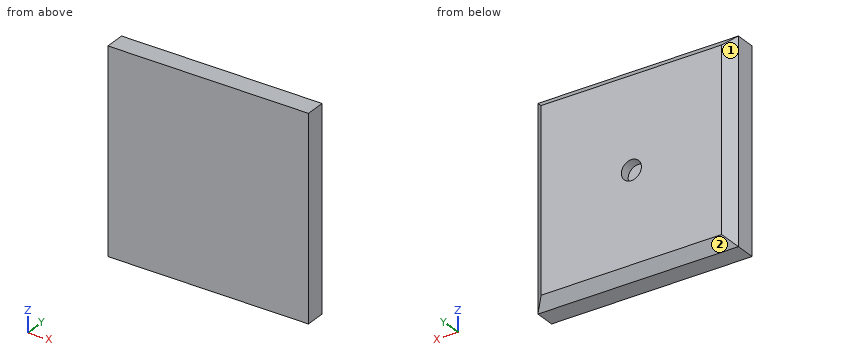
from build123d import *

# Parameters (mm, degrees)
CROQUIS1_W              = 100
CROQUIS1_H              = 100
SALIENTE_EXTRUIR1_DEPTH = 15
CHAFL_N1_SIZE           = 5
CROQUIS3_R              = 5
CORTAR_EXTRUIR1_DEPTH   = 5


with BuildPart() as part:
    # Croquis1 → Saliente-Extruir1 (new body)
    with BuildSketch(Plane(origin=(0, 0, 0), x_dir=(1, 0, 0), z_dir=(0, 1, 0))):
        with Locations((50, 50)):
            Rectangle(CROQUIS1_W, CROQUIS1_H)
    extrude(amount=SALIENTE_EXTRUIR1_DEPTH)

    # Chaflán1
    chafl_n1_edges = [part.edges().sort_by_distance(p)[0] for p in [
        (100, 15, -50),
        (50, 15, -100),
        (0, 15, -50),
        (50, 15, 0),
    ]]
    chamfer(chafl_n1_edges, length=CHAFL_N1_SIZE)

    # Croquis3 → Cortar-Extruir1 (cut)
    with BuildSketch(Plane(origin=(0, 15, 0), x_dir=(1, 0, 0), z_dir=(0, 1, 0))):
        with Locations(Location((50, 50, 0), (0, 0, 270))):
            Circle(CROQUIS3_R)
    extrude(amount=-CORTAR_EXTRUIR1_DEPTH, mode=Mode.SUBTRACT)


solid = part.part
Could you check a few things on this model? Use its own coordinates, in mm. Face numbers are marked on the shaded views. Round coordinates to 2 decimals unless told otherwise and drop trailing zeros. Order: outer loops, then holes, each group sorted by start corner. A loop starts at its lowest first (then second) coordinate and runs counter-clockwise, first axis right, second up. Notation, with made-up numbers: M 0.5,-32.75 L 46.5,-32.75 A30 cw 46.5,4.25 Z; hole C 58,0 d10. An arc over 180 degrees is marked long. One line per item, written item: value.
(1) Imagine slicing it at A-A (y = 13). Write out the boundary of the cut face in (x, z), and give its area (3 significant figures).
Ans:
outline: M 3,-97 L 97,-97 L 97,-3 L 3,-3 Z; hole C 50,-50 d10
area: 8,760 mm^2
(2) Imagine slicing it at D-D (x = 66.5). Write out the boundary of the cut face in (y, z), and give its area (4 significant figures).
Ans:
outline: M 0,-100 L 10,-100 L 15,-95 L 15,-5 L 10,0 L 0,0 Z
area: 1,475 mm^2
(3) I need wall thicknesses on line 1 along X through (y, z) = (11.8, -50); line 2 along X through (y, z) = (12.15, -50); line 3 along X through (y, z) = (12, -11). Which ranges of each line are inside material? Lowest first, please. Write a range as from..to.
Ans:
line 1: x = 1.8..45, 55..98.2
line 2: x = 2.15..45, 55..97.85
line 3: x = 2..98
(4) I'm going to push a flat-ended pin straight in: P1, Ø2, axis at y = 12.5, z = -23, coming from the +X side. Where does the tip first touch, or does it pass through?
Ans:
P1: stops at x = 98.5
(5) Imagine slicing it at B-B (z = -50). Write out the boundary of the cut face in (x, y), and give its area (4 significant figures).
Ans:
outline: M 0,0 L 100,0 L 100,10 L 95,15 L 55,15 L 55,10 L 45,10 L 45,15 L 5,15 L 0,10 Z
area: 1,425 mm^2
(6) If we mould it in two halves opening along Z, with no side actions, what happens to the marked faces 1 and 2? For each: released by +Z, released by -Z, zero draft, split by the parting line, or undercut.
Ans:
face 1: zero draft
face 2: released by -Z
(7) Imagine slicing it at C-C (x = 50). Write out the boundary of the cut face in (y, z), and give its area (4 significant figures).
Ans:
outline: M 0,-100 L 10,-100 L 15,-95 L 15,-55 L 10,-55 L 10,-45 L 15,-45 L 15,-5 L 10,0 L 0,0 Z
area: 1,425 mm^2
